Here's how the part is built. I have some questions about the finished solid (model axes, mm). A direction names the side the tool comes from. Give positions to 0.01 mm unless a question says otherwise; leave off trailing zeros. Loops run counter-clockwise (first coordinate to the right, second up) from the corner with the lowest first, then second, coordinate; pieces in that order, holes last. Notation, with made-up numbers: M 60,52 L 114,52 A23 cw 114,60 Z; hole C -35.5,34 d4. An arc over 180 degrees is marked long. Answer as CSV lines item,"result". Start each with the question number.
Item 1: I want a section at B-B on x = -43. List the corners of the cut face in (y, z) for me.
Item 2: If I drill on line 1 along Y through (x, z) = (-2.5, 41); line 2 along X through (y, z) = (20, 3); line 3 along Z through (x, y) = (-23, 13), over which ranges is the centre line in solid material (lowest first)? Write a range as from..to.
Item 3: I want a section at C-C on y = 7. List the corners of the cut face in (x, z) for me.
Item 4: For faces 1 (the flat face through (-35, 30, 20)), 2 (the flat face through (20, 15, 20)), 3 (the flat face through (43, 35, 20)), 4 (the cylindrical face through (-48, 7, 20)), 5 (the cylindrical face through (37.48, 25.35, -14.38)), which set-ups out of +Z, -Z, +X, -X, +Y, -Y let a thin tool reach every point of the face, with its end or its side?
Item 5: I want a section at D-D on x = -7. List the corners of the cut face in (y, z) for me.
Item 6: If we mould it in two halves opening along X, with no side actions, what happens to faces 6 (the flat face through (-15, 8, 60)), 7 (the cylindrical face through (36.94, 25.35, 54.76)), 8 (the flat face through (-20, 15, 20))? For each: released by +X, released by -X, zero draft, split by the parting line, or undercut.
Item 7: Will these pins go through, and if not, where does the flat tip stop? P1, Ø3, axis at x = 43, z = 18.5, coming from the -Y side; P2, Ø22.5, axis at x = 37.5, y = 21, coming from the -Z side; P3, Ø15, axis at y = 16, z = 24.5, coming from the -X side.
from build123d import *

# Parameters (mm, degrees)
SKETCH_1_W          = 100
SKETCH_1_H          = 40
EXTRUDE_1_DEPTH     = 80
SKETCH_3_W          = 30
SKETCH_3_H          = 30
CUT_EXTRUDE_2_DEPTH = 20
SKETCH_6_R          = 5
EXTRUDE_2_DEPTH     = 20
SKETCH_7_W          = 70
SKETCH_7_H          = 80
CUT_EXTRUDE_3_DEPTH = 40
FILLET_1_R          = 30
FILLET_2_R          = 30
FILLET_3_R          = 30
FILLET_4_R          = 20
FILLET_5_R          = 20
SKETCH1_R           = 5
CUT_EXTRUDE1_DEPTH  = 5


with BuildPart() as part:
    # 草圖1 → 填料-伸長1 (new body)
    with BuildSketch(Plane(origin=(0, 0, 0), x_dir=(1, 0, 0), z_dir=(0, 1, 0))):
        Rectangle(SKETCH_1_W, SKETCH_1_H)
    extrude_1 = extrude(amount=EXTRUDE_1_DEPTH)

    # 草圖3 → 除料-伸長2 (cut)
    with BuildSketch(Plane.XY.offset(20)):
        with Locations((-35, 15)):
            Rectangle(SKETCH_3_W, SKETCH_3_H)
        with Locations((35, 15)):
            Rectangle(SKETCH_3_W, SKETCH_3_H)
    cut_extrude_2 = extrude(amount=-CUT_EXTRUDE_2_DEPTH, mode=Mode.SUBTRACT)

    # 草圖6 → 填料-伸長2 (add)
    with BuildSketch(Plane.XY):
        with Locations((-43, 7)):
            Circle(SKETCH_6_R)
    extrude_2 = extrude(amount=EXTRUDE_2_DEPTH)

    # 鏡射3: 填料-伸長1, 除料-伸長2, 填料-伸長2 across plane
    add(extrude_1.mirror(Plane(origin=(-50, 80, 20), x_dir=(1, 0, 0), z_dir=(0, 0, -1))))
    add(cut_extrude_2.mirror(Plane(origin=(-50, 80, 20), x_dir=(1, 0, 0), z_dir=(0, 0, -1))), mode=Mode.SUBTRACT)
    add(extrude_2.mirror(Plane(origin=(-50, 80, 20), x_dir=(1, 0, 0), z_dir=(0, 0, -1))))

    # 草圖7 → 除料-伸長3 (cut)
    with BuildSketch(Plane(origin=(0, 80, 0), x_dir=(1, 0, 0), z_dir=(0, 1, 0))):
        with Locations((-15, -20)):
            Rectangle(SKETCH_7_W, SKETCH_7_H)
    extrude(amount=-CUT_EXTRUDE_3_DEPTH, mode=Mode.SUBTRACT)

    # 圓角1
    fillet_1_edges = [part.edges().sort_by_distance(p)[0] for p in [
        (50, 80, 20),
    ]]
    fillet(fillet_1_edges, radius=FILLET_1_R - 0.0001)  # a hair under: the kernel refuses the full size

    # 圓角2
    fillet_2_edges = [part.edges().sort_by_distance(p)[0] for p in [
        (50, 25.00005, 60),
        (41.213232725, 71.213232725, 60),
    ]]
    fillet(fillet_2_edges, radius=FILLET_2_R - 0.0001)  # a hair under: the kernel refuses the full size

    # 圓角3
    fillet_3_edges = [part.edges().sort_by_distance(p)[0] for p in [
        (50, 25.00005, -20),
        (41.213232725, 71.213232725, -20),
    ]]
    fillet(fillet_3_edges, radius=FILLET_3_R - 0.0001)  # a hair under: the kernel refuses the full size

    # 圓角4
    fillet_4_edges = [part.edges().sort_by_distance(p)[0] for p in [
        (-15, 40, 60),
    ]]
    fillet(fillet_4_edges, radius=FILLET_4_R)

    # 圓角5
    fillet_5_edges = [part.edges().sort_by_distance(p)[0] for p in [
        (-15, 40, -20),
    ]]
    fillet(fillet_5_edges, radius=FILLET_5_R)

    # Sketch1 → Cut-Extrude1 (cut)
    with BuildSketch(Plane.XZ.offset(-30)):
        with Locations((43, 20)):
            Circle(SKETCH1_R)
    extrude(amount=-CUT_EXTRUDE1_DEPTH, mode=Mode.SUBTRACT)


solid = part.part
Result:
1,outline,"M 0,-20 L 20,-20 A20 ccw 40,0 L 40,40 A20 ccw 20,60 L 0,60 L 0,40 L 2,40 L 2,0 L 0,0 Z; hole M 12,0 L 30,0 L 30,40 L 12,40 Z"
2,line 1,"0..39.97"
2,line 2,"-20..20"
2,line 3,"-20..0, 40..60"
3,outline,"M -50,-20 L 20,-20 A30 ccw 48.28,0 L 20,0 L 20,40 L 48.28,40 A30 ccw 20,60 L -50,60 L -50,40 L -48,40 L -48,0 L -50,0 Z; hole M -38,0 L -20,0 L -20,40 L -38,40 Z"
4,face 1,"-X"
4,face 2,"+X, -Y"
4,face 3,"-Y"
4,face 4,"none"
4,face 5,"-Z, +X, +Y, -Y"
5,outline,"M 0,-20 L 20,-20 A20 ccw 40,0 L 40,40 A20 ccw 20,60 L 0,60 Z"
6,face 6,"zero draft"
6,face 7,"released by +X"
6,face 8,"undercut"
7,P1,"y = 35"
7,P2,"z = -19.34"
7,P3,"x = -47.77"
